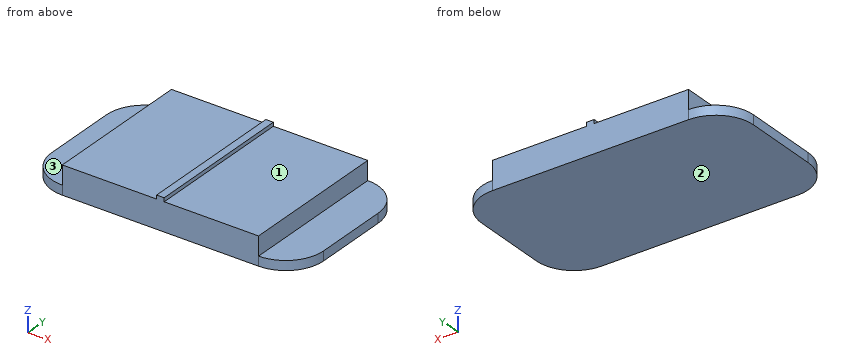
from build123d import *

# Parameters (mm, degrees)
EXTRUDE_1_DEPTH = 40
FILLET_3_R      = 10
FILLET_6_R      = 10
FILLET_7_R      = 10
FILLET_8_R      = 10


with BuildPart() as part:
    # Эскиз1 → Бобышка-Вытянуть1 (new body)
    with BuildSketch(Plane(origin=(0, 0, 0), x_dir=(1, 0, 0), z_dir=(0, 1, 0))):
        Polygon((-26, -14.521028037), (-26, -9.521028037), (-32, -9.521028037), (-36, -9.521028037), (-36, -7.021028037), (-1, -7.021028037), (1, -7.021028037), (36, -7.021028037), (36, -9.521028037), (32, -9.521028037), (26, -9.521028037), (26, -14.521028037), (1, -14.521028037), (1, -15.521028037), (-1, -15.521028037), (-1, -14.521028037), align=None)
    extrude(amount=EXTRUDE_1_DEPTH)

    # Скругление3
    fillet_3_edges = [part.edges().sort_by_distance(p)[0] for p in [
        (-36, 40, 8.271028037),
    ]]
    fillet(fillet_3_edges, radius=FILLET_3_R)

    # Скругление6
    fillet_6_edges = [part.edges().sort_by_distance(p)[0] for p in [
        (-36, 0, 8.271028037),
    ]]
    fillet(fillet_6_edges, radius=FILLET_6_R)

    # Скругление7
    fillet_7_edges = [part.edges().sort_by_distance(p)[0] for p in [
        (36, 40, 8.271028037),
    ]]
    fillet(fillet_7_edges, radius=FILLET_7_R)

    # Скругление8
    fillet_8_edges = [part.edges().sort_by_distance(p)[0] for p in [
        (36, 0, 8.271028037),
    ]]
    fillet(fillet_8_edges, radius=FILLET_8_R)


solid = part.part
Check sheet for the modelled part. Datum: model origin and axes. Units: mm. Face numbers are marked on the shaded views. A direction names the side the tool comes from. Round coordinates to 2 decimals unless told otherwise and drop trailing zeros. Order: outer loops, then holes, each group sorted by start corner. A loop starts at its lowest first (then second) coordinate and runs counter-clockwise, first axis right, second up. Notation, with made-up numbers: M -25,-7.5 L -20,-7.5 A13 cw -20,-1.5 Z; hole C -16.75,-37.75 d2. An arc over 180 degrees is marked long. One line per item, written item: value. Start each with the question number.
1. Scan lines: line 1 along Z through (x, y) = (23.5, 32); line 2 along X through (y, z) = (10, 12); line 3 along Z through (x, y) = (33.5, 27). Record each from-to range of solid material in increasing order.
2. Section check B-B on y = 4. Enter the section's corners in (x, z), and give its area (3 significant figures).
3. Access from +Z, -Z, +X, -X, +Y, -Y to the whole of each face (thin tool, end or side, straight path). Record for the marked faces 1, 2 and 3.
4. Section check C-C on x = -16. Enter the section's corners in (y, z), and give its area (3 significant figures).
5. Section check D-D on y = 22.5. Enter the section's corners in (x, z).
6. Gauge pin test, flat ends, axial feed: P1, Ø20, axis at x = -12, y = 28, coming from the +Z side; P2, Ø11, axis at x = -32, y = 25, coming from the +Z side; P3, Ø4, axis at y = 23.5, z = 10.5, coming from the -X side; P4, Ø1.5, axis at y = 16, z = 13, coming from the +X side. Record the tip position at first contact, or that the pin passes through.
7. Section check A-A on z = 8. Enter the section's corners in (x, y), and give its area (3 significant figures).
Results found:
1. line 1: 7.02 to 14.52
1. line 2: -26 to 26
1. line 3: 7.02 to 9.52
2. outline: M -34,7.02 L 34,7.02 L 34,9.52 L 26,9.52 L 26,14.52 L 1,14.52 L 1,15.52 L -1,15.52 L -1,14.52 L -26,14.52 L -26,9.52 L -34,9.52 Z
2. area: 432 mm^2
3. face 1: +Z, +X, +Y, -Y
3. face 2: -Z, +X, -X, +Y, -Y
3. face 3: +Z, -X, +Y, -Y
4. outline: M 0,7.02 L 40,7.02 L 40,14.52 L 0,14.52 Z
4. area: 300 mm^2
5. outline: M -36,7.02 L 36,7.02 L 36,9.52 L 26,9.52 L 26,14.52 L 1,14.52 L 1,15.52 L -1,15.52 L -1,14.52 L -26,14.52 L -26,9.52 L -36,9.52 Z
6. P1: z = 14.52
6. P2: z = 9.52
6. P3: x = -36
6. P4: x = 26
7. outline: M -36,10 A10 ccw -26,0 L 26,0 A10 ccw 36,10 L 36,30 A10 ccw 26,40 L -26,40 A10 ccw -36,30 Z
7. area: 2,790 mm^2
